```python
from build123d import *

# Parameters (mm, degrees)
BOSS_EXTRUDE1_DEPTH = 13
CUT_EXTRUDE3_DEPTH  = 14
FILLET2_R           = 0.3
FILLET1_R           = 0.8
SKETCH3_OUTSIDE_W   = 154.491
SKETCH3_OUTSIDE_H   = 40.548
SKETCH3_OUTSIDE_W_2 = 5.910380326
SKETCH3_OUTSIDE_H_2 = 7.5
CUT_EXTRUDE2_DEPTH  = 35


with BuildPart() as part:
    # Sketch1 → Boss-Extrude1 (new body)
    with BuildSketch(Plane(origin=(0, 0, 0), x_dir=(1, 0, 0), z_dir=(0, 1, 0))):
        with BuildLine():
            Line((0, 51.7), (0, 53))
            ThreePointArc((0, 53), (-4, 49), (0, 45))
            ThreePointArc((0, 45), (43.466662183, 11.64685703), (22.5, -38.97114317))
            Line((22.5, -38.97114317), (-7.810889132, -56.47114317))
            Line((-7.810889132, -56.47114317), (-5.810889132, -59.935244785))
            Line((-5.810889132, -59.935244785), (24.5, -42.435244785))
            ThreePointArc((24.5, -42.435244785), (47.509263839, -11.994575836), (41.707047143, 25.720074234))
            ThreePointArc((41.707047143, 25.720074234), (25.051905135, 42.111780407), (2.698975076, 48.925612245))
            ThreePointArc((2.698975076, 48.925612245), (-1.935309657, 47.117295421), (0, 51.7))
        make_face()
        with BuildLine():
            Line((51.921017872, 32.018867925), (0, 53))
            Line((0, 53), (0, 51.7))
            ThreePointArc((0, 51.7), (1.909188309, 50.909188309), (2.7, 49))
            ThreePointArc((2.7, 49), (2.699743757, 48.962802592), (2.698975076, 48.925612245))
            ThreePointArc((2.698975076, 48.925612245), (25.051905135, 42.111780407), (41.707047143, 25.720074234))
            Line((41.707047143, 25.720074234), (51.921017872, 32.018867925))
        make_face()
    extrude(amount=BOSS_EXTRUDE1_DEPTH)

    # Sketch2 → Cut-Extrude3 (cut, through all)
    with BuildSketch(Plane(origin=(0, 13, 0), x_dir=(1, 0, 0), z_dir=(0, 1, 0))):
        Polygon((-5.844863729, -57.876399059), (-4.944863729, -59.435244785), (-2.346787517, -57.935244785), align=None)
        Polygon((-3.246787517, -56.376399059), (-2.346787517, -57.935244785), (0.251288694, -56.435244785), align=None)
        Polygon((-0.648711306, -54.876399059), (0.251288694, -56.435244785), (2.849364905, -54.935244785), align=None)
        Polygon((1.949364905, -53.376399059), (2.849364905, -54.935244785), (5.447441117, -53.435244785), align=None)
        Polygon((4.547441117, -51.876399059), (5.447441117, -53.435244785), (8.045517328, -51.935244785), align=None)
        Polygon((7.145517328, -50.376399059), (8.045517328, -51.935244785), (10.643593539, -50.435244785), align=None)
        Polygon((9.743593539, -48.876399059), (10.643593539, -50.435244785), (13.241669751, -48.935244785), align=None)
        Polygon((12.341669751, -47.376399059), (13.241669751, -48.935244785), (15.839745962, -47.435244785), align=None)
        Polygon((14.939745962, -45.876399059), (15.839745962, -47.435244785), (18.437822174, -45.935244785), align=None)
        Polygon((17.537822174, -44.376399059), (18.437822174, -45.935244785), (21.035898385, -44.435244785), align=None)
        Polygon((20.135898385, -42.876399059), (21.035898385, -44.435244785), (23.633974596, -42.935244785), align=None)
    extrude(amount=-CUT_EXTRUDE3_DEPTH, mode=Mode.SUBTRACT)

    # Fillet2
    fillet2_edges = [part.edges().sort_by_distance(p)[0] for p in [
        (-3.246787517, 6.5, 56.376399059),
        (0.251288694, 6.5, 56.435244785),
        (1.949364905, 6.5, 53.376399059),
        (5.447441117, 6.5, 53.435244785),
        (7.145517328, 6.5, 50.376399059),
        (10.643593539, 6.5, 50.435244785),
        (12.341669751, 6.5, 47.376399059),
        (15.839745962, 6.5, 47.435244785),
        (17.537822174, 6.5, 44.376399059),
        (21.035898385, 6.5, 44.435244785),
        (-5.810889132, 6.5, 59.935244785),
        (-5.844863729, 6.5, 57.876399059),
        (-2.346787517, 6.5, 57.935244785),
        (-4.944863729, 6.5, 59.435244785),
        (-0.648711306, 6.5, 54.876399059),
        (2.849364905, 6.5, 54.935244785),
        (4.547441117, 6.5, 51.876399059),
        (8.045517328, 6.5, 51.935244785),
        (9.743593539, 6.5, 48.876399059),
        (13.241669751, 6.5, 48.935244785),
        (14.939745962, 6.5, 45.876399059),
        (18.437822174, 6.5, 45.935244785),
        (20.135898385, 6.5, 42.876399059),
    ]]
    fillet(fillet2_edges, radius=FILLET2_R)

    # Fillet1
    fillet1_edges = [part.edges().sort_by_distance(p)[0] for p in [
        (51.921017872, 6.5, -32.018867925),
        (41.707047143, 6.5, -25.720074234),
        (-7.810889132, 6.5, 56.47114317),
        (0, 6.5, -53),
    ]]
    fillet(fillet1_edges, radius=FILLET1_R)

    # Sketch3 outside → Cut-Extrude2 (cut)
    with BuildSketch(Plane(origin=(-30.310889132, 0, 17.5), x_dir=(0.5, 0, 0.866025404), z_dir=(-0.866025404, 0, 0.5))):
        with Locations((13.8165, 6.5)):
            Rectangle(SKETCH3_OUTSIDE_W, SKETCH3_OUTSIDE_H)
        with Locations((47.141631591, 6.5)):
            Rectangle(SKETCH3_OUTSIDE_W_2, SKETCH3_OUTSIDE_H_2, mode=Mode.SUBTRACT)
    extrude(amount=-CUT_EXTRUDE2_DEPTH, mode=Mode.SUBTRACT)


solid = part.part
```
Source: CAD feature listing. Evaluate the final solid. Frame: model axes, mm. A direction names the side the tool comes from. Give positions to 0.01 mm unless a question says otherwise; leave off trailing zeros. Loops run counter-clockwise (first coordinate to the right, second up) from the corner with the lowest first, then second, coordinate; pieces in that order, holes last. Notation, with made-up numbers: (-10, -29.75) -> (7, -29.75) arc R11 ccw to (7, -9.75) -> close; hole circle Ø4 at (73, 87). An arc over 180 degrees is marked (long way). Put each result on its own line as item: value. Start each with the question number.
1) Material intervals for probe 1 along Z at (x, y) = (18, 9.25); probe 2 along X at (y, z) = (4.25, -49); probe 3 along Z at (x, y) = (31.5, 6.75), sorted ascending.
2) Contact query for flat-ended pins moving along their axis: P1, Ø1.5, axis at x = 41.5, z = 12, coming from the +Y side; P2, Ø5, axis at x = 28, y = 10, coming from the -Z side; P3, Ø23, axis at x = 11.5, z = 46, coming from the -Y side; P4, Ø10.5, axis at x = 8.5, z = 44.5, coming from the +Y side. Output: stop coordinate, or through.
3) Cut plane C-C (z = -22.5). Return loops of the section in (x, y), then the cut area to 3 significant figures.
4) Cut plane B-B (z = 6). Return loops of the section in (x, y).
5) Reachability of faces 1 (the face through (23.5, 1.4, 40.7)), 2 (the face through (42, 0, -20)), 3 (the face through (23.5, 11.6, 40.7)), 4 (the face through (7.9, 6.4, 47.4)) from +Z, -Z, +X, -X, +Y, -Y: full face, straight path, thin tool, end or side. Return the list, or none.
6) Cut plane A-A (x = 32.5). Return loops of the section in (y, z), then the cut area to 3 significant figures.
Results are:
1. probe 1: z = -45.73 to -41.24, 41.57 to 44.39, 45.18 to 45.91
1. probe 2: x = -4 to -2.7, 2.7 to 9.9
1. probe 3: z = -40.27 to -32.14, 32.14 to 37.53
2. P1: passes through
2. P2: stops at z = -42.7
2. P3: stops at y = 2.75
2. P4: stops at y = 10.25
3. outline: (38.97, 0) -> (43.53, 0) -> (43.53, 13) -> (38.97, 13) -> close
3. area: 59.2 mm2
4. outline: (44.6, 0) -> (48.63, 0) -> (48.63, 13) -> (44.6, 13) -> close
5. face 1: +Z, -X, -Y
5. face 2: +Z, -Z, +X, -X, -Y
5. face 3: +Z, -X, +Y
5. face 4: -X, +Y, -Y
6. outline: (0, -39.87) -> (13, -39.87) -> (13, -31.12) -> (0, -31.12) -> close; (0, 31.12) -> (13, 31.12) -> (13, 36.67) -> (0, 36.67) -> close
6. area: 186 mm2
